Could you check a few things on this model? Use its own coordinates, in mm. A direction names the side the tool comes from. Coordinates: 2 decimals unless noted, no trailing zeros. Order: outer loops, then holes, each group sorted by start corner. A loop starts at its lowest first (then second) coordinate and runs counter-clockwise, first axis right, second up. Notation, with made-up numbers: (30.5, 34.25) - (61.5, 34.25) arc R13 ccw to (61.5, 39.25) - close; hole circle Ø11 at (81, 7.25). An arc over 180 degrees is marked (long way). One line per item, written item: value. Start each with the question number.
from build123d import *

# Parameters (mm, degrees)
F0_W      = 25.4
F0_H      = 25.4
F1_DEPTH  = 622.3
F2_W      = 25.4
F2_H      = 25.4
F3_DEPTH  = 622.3
F4_W      = 25.4
F4_H      = 25.4
F5_DEPTH  = 622.3
F6_W      = 25.4
F6_H      = 25.4
F7_DEPTH  = 622.3
F9_DEPTH  = 12.7
F10_DEPTH = 12.7
F11_W     = 25.4
F11_H     = 25.4
F12_DEPTH = 1079.5
F14_DEPTH = 12.7
F15_DEPTH = 12.7
F17_DEPTH = 12.7
F18_DEPTH = 12.7
F19_ANGLE = 90
F21_ANGLE = 180


with BuildPart() as f1:
    # F0 (on Front) → F1 (new body)
    with BuildSketch(Plane.XZ):
        Rectangle(F0_W, F0_H)
    extrude(amount=F1_DEPTH)

    # F2 (on Front) → F3 (join)
    with BuildSketch(Plane.XZ):
        Rectangle(F2_W, F2_H)
    extrude(amount=-F3_DEPTH)

    # F4 (on Top) → F5 (join)
    with BuildSketch(Plane.XY):
        Rectangle(F4_W, F4_H)
    extrude(amount=-F5_DEPTH)



with BuildPart() as f7:
    # F6 (on Top) → F7 (new body)
    with BuildSketch(Plane.XY):
        Rectangle(F6_W, F6_H)
    extrude(amount=F7_DEPTH)


with BuildPart() as f1_1:
    add(f1.part)

    add(f7.part)  # F9 merges F7
    # F8 (on Right) → F9 (join)
    with BuildSketch(Plane.YZ):
        Polygon((12.7, 317.5), (317.4895992739, 10.1820296971), (353.2631639393, 10.1820296971), (352.6753836214, 10.7746859253), (317.529985282, 10.7746859253), (12.7403860081, 318.0926562282), (12.7403860081, 353.5296019405), (12.7, 353.5703229692), align=None)
        Polygon((317.529985282, 10.7746859253), (352.6753836214, 10.7746859253), (12.7403860081, 353.5296019405), (12.7403860081, 318.0926562282), align=None)
        Polygon((12.7403860081, 353.5296019405), (352.6753836214, 10.7746859253), (353.3035499474, 10.7746859253), (12.7403860081, 354.1629791974), align=None)
        Polygon((-352.787982248, -12.7), (-317.5, -12.7), (-12.7, -317.5), (-12.7, -352.787982248), (-12.6596139919, -352.8283682561), (-12.6596139919, -316.9073437718), (-317.4596139919, -12.1073437718), (-353.3806384762, -12.1073437718), align=None)
        Polygon((-12.7, -317.5), (-317.5, -12.7), (-352.787982248, -12.7), (-12.7, -352.787982248), align=None)
        Polygon((-12.7, -352.787982248), (-352.787982248, -12.7), (-353.4210244843, -12.7), (-12.7, -353.4210244843), align=None)
    extrude(amount=F9_DEPTH)

    # F8 (on Right) → F10 (join)
    with BuildSketch(Plane.YZ):
        Polygon((12.7, 317.5), (317.4895992739, 10.1820296971), (353.2631639393, 10.1820296971), (352.6753836214, 10.7746859253), (317.529985282, 10.7746859253), (12.7403860081, 318.0926562282), (12.7403860081, 353.5296019405), (12.7, 353.5703229692), align=None)
        Polygon((317.529985282, 10.7746859253), (352.6753836214, 10.7746859253), (12.7403860081, 353.5296019405), (12.7403860081, 318.0926562282), align=None)
        Polygon((12.7403860081, 353.5296019405), (352.6753836214, 10.7746859253), (353.3035499474, 10.7746859253), (12.7403860081, 354.1629791974), align=None)
        Polygon((-352.787982248, -12.7), (-317.5, -12.7), (-12.7, -317.5), (-12.7, -352.787982248), (-12.6596139919, -352.8283682561), (-12.6596139919, -316.9073437718), (-317.4596139919, -12.1073437718), (-353.3806384762, -12.1073437718), align=None)
        Polygon((-12.7, -317.5), (-317.5, -12.7), (-352.787982248, -12.7), (-12.7, -352.787982248), align=None)
        Polygon((-12.7, -352.787982248), (-352.787982248, -12.7), (-353.4210244843, -12.7), (-12.7, -353.4210244843), align=None)
    extrude(amount=-F10_DEPTH)

    # F11 (on Right) → F12 (join)
    with BuildSketch(Plane.YZ):
        Rectangle(F11_W, F11_H)
    extrude(amount=F12_DEPTH)

    # F13 (on Front) → F14 (join)
    with BuildSketch(Plane.XZ):
        Polygon((12.7, 349.2973023653), (12.7, 317.5), (469.9, 12.7), (515.6905011984, 12.7), align=None)
        Polygon((515.6905011984, -12.7), (469.9, -12.7), (12.7, -317.5), (12.7, -348.0270007989), align=None)
    extrude(amount=F14_DEPTH)

    # F13 (on Front) → F15 (join)
    with BuildSketch(Plane.XZ):
        Polygon((12.7, 349.2973023653), (12.7, 317.5), (469.9, 12.7), (515.6905011984, 12.7), align=None)
        Polygon((515.6905011984, -12.7), (469.9, -12.7), (12.7, -317.5), (12.7, -348.0270007989), align=None)
    extrude(amount=-F15_DEPTH)

    # F16 (on Top) → F17 (join)
    with BuildSketch(Plane.XY):
        Polygon((12.7, 317.5), (469.9, 12.7), (515.6905011984, 12.7), (12.7, 348.0270007989), align=None)
        Polygon((515.6905011984, -12.7), (469.9, -12.7), (12.7, -317.5), (12.7, -348.0270007989), align=None)
    extrude(amount=F17_DEPTH)

    # F16 (on Top) → F18 (join)
    with BuildSketch(Plane.XY):
        Polygon((12.7, 317.5), (469.9, 12.7), (515.6905011984, 12.7), (12.7, 348.0270007989), align=None)
        Polygon((515.6905011984, -12.7), (469.9, -12.7), (12.7, -317.5), (12.7, -348.0270007989), align=None)
    extrude(amount=-F18_DEPTH)


with BuildPart() as f1_2:
    # F19: moved
    add(f1_1.part.rotate(Axis((-12.7, -311.15, -12.7), (0, 1, 0)), F19_ANGLE))


with BuildPart() as f1_3:
    # F20: moved
    add(f1_2.part.moved(Location((0, 0, -25.4))))


with BuildPart() as f1_4:
    # F21: moved
    add(f1_3.part.rotate(Axis((311.15, 12.7, -38.1), (-1, 0, 0)), F21_ANGLE))


with BuildPart() as f1_5:
    # F22: moved
    add(f1_4.part.moved(Location((0, -25.4, 0))))


with BuildPart() as f1_6:
    # F23: moved
    add(f1_5.part.moved(Location((0, 0, 25.4))))


solid = f1_6.part
Q1. I want a section at D-D on z = 498.5. Please give me the cut outline in (x, y).
Q2. I want a section at C-C on y = 125.5. Please give me the cut outline in (x, z).
Q3. We'd pull the mould along X, two halves only. Please class faces 1 (the flat face through (-162.966, -0.178, 244.5)), 2 (the flat face through (-12.7, -251, 133)), 3 (the flat face through (-0.178, 162.966, 244.5)): +X half, -X half, draft (parallel to the pull), parting line (faces both ways), or undercut.
Q4. I want a section at B-B on z = 180. Please give me the cut outline in (x, y).
Q5. Which directions (+Z, -Z, +X, -X, +Y, -Y) give clear straight access to the entire face, cutting with the end or side of a thin tool? Please do faces 4 (the flat face through (248, 12.7, 133)), 5 (the flat face through (-166.913, 162.654, -0.178)), 6 (the flat face through (0.178, -167.234, 238.1)), 7 (the flat face through (167.234, 0.178, 238.1)).
Q6. If I drill on L1, parallel to X at y = 2.5, z = 907.5; L2, parallel to X at y = 10.5, z = 166; L3, parallel to Z at x = -282.5, y = 10, over which ranges is the centre line in solid material (lowest first)?
Q7. I want a section at A-A on x = 41. Please give me the cut outline in (y, z), then the cut area to 3 significant figures.
Q8. I'm going to push flat-ended pins straight in: pin 1 (0.7 mm diameter, centred on x = 354, z = 6.5, fed in from +Y); pin 2 (12.5 mm diameter, centred on y = 4, z = 930, fed in from +X); pin 3 (12.5 mm diameter, centred on x = 208.5, z = 5, fed in from -Y). Where does each tip first touch, or does it pass through?
Values follow:
1. outline: (-24.16, -12.7) - (-12.7, -12.7) - (-12.7, -24.16) - (12.7, -24.16) - (12.7, -12.7) - (24.2, -12.7) - (24.2, 12.7) - (12.7, 12.7) - (12.7, 24.16) - (-12.7, 24.16) - (-12.7, 12.7) - (-24.16, 12.7) - close
2. outline: (-240.62, -12.7) - (-204.07, -12.7) - (-204.07, 12.7) - (-240.62, 12.7) - close; (-12.7, -12.7) - (12.7, -12.7) - (12.7, 12.7) - (-12.7, 12.7) - close; (-12.7, 300.7) - (12.7, 300.7) - (12.7, 346.49) - (-12.7, 346.49) - close
3. face 1: undercut
3. face 2: -X half
3. face 3: draft
4. outline: (-236.49, -12.7) - (-205.97, -12.7) - (-205.97, 12.7) - (-236.49, 12.7) - close; (-12.7, -236.49) - (12.7, -236.49) - (12.7, -205.97) - (-12.7, -205.97) - close; (-12.7, -12.7) - (12.7, -12.7) - (12.7, 12.7) - (-12.7, 12.7) - close; (-12.7, 205.97) - (12.7, 205.97) - (12.7, 236.49) - (-12.7, 236.49) - close; (205.97, -12.7) - (237.34, -12.7) - (237.34, 12.7) - (205.97, 12.7) - close
5. face 4: +Z, -Z, +X, +Y
5. face 5: +Z, -Z
5. face 6: +X, -X
5. face 7: +Y, -Y
6. L1: x = -12.7 to 12.7
6. L2: x = -245.83 to -215.3, -12.7 to 12.7, 215.3 to 246.71
6. L3: z = -12.7 to 12.7, 65.2 to 110.99
7. outline: (-323.33, -12.7) - (-286.93, -12.7) - (-286.93, 12.7) - (-323.33, 12.7) - close; (-12.7, -12.7) - (12.7, -12.7) - (12.7, 12.7) - (-12.7, 12.7) - close; (-12.7, 427.45) - (12.7, 427.45) - (12.7, 473.4) - (-12.7, 473.4) - close
7. area: 2,740 mm^2
8. pin 1: stops at y = 12.7
8. pin 2: stops at x = 12.7
8. pin 3: stops at y = -163.4
